```python
from build123d import *

# Parameters (mm, degrees)
SKETCH1_R           = 7.4
BOSS_EXTRUDE1_DEPTH = 6
SKETCH2_R           = 10
SKETCH2_R_2         = 1.5
BOSS_EXTRUDE2_DEPTH = 3
FILLET1_R           = 2.5


with BuildPart() as part:
    # Sketch1 → Boss-Extrude1 (new body)
    with BuildSketch(Plane(origin=(0, 0, 0), x_dir=(1, 0, 0), z_dir=(0, 1, 0))):
        with Locations(Location((0, 0, 0), (0, 0, 270))):
            Circle(SKETCH1_R)
        with BuildLine():
            Line((2.2, 2.219374912), (2.2, -2.219374912))
            ThreePointArc((2.2, -2.219374912), (-3.125, 0), (2.2, 2.219374912))
        make_face(mode=Mode.SUBTRACT)
    extrude(amount=BOSS_EXTRUDE1_DEPTH)

    # Sketch2 → Boss-Extrude2 (add)
    with BuildSketch(Plane(origin=(0, 6, 0), x_dir=(1, 0, 0), z_dir=(0, 1, 0))):
        with Locations(Location((0, 0, 0), (0, 0, 270))):
            Circle(SKETCH2_R)
        with Locations(Location((0, 0, 0), (0, 0, 270))):
            Circle(SKETCH2_R_2, mode=Mode.SUBTRACT)
    extrude(amount=BOSS_EXTRUDE2_DEPTH)

    # Fillet1
    fillet1_edges = [part.edges().sort_by_distance(p)[0] for p in [
        (0, 9, -10),
    ]]
    fillet(fillet1_edges, radius=FILLET1_R)


solid = part.part
```
The model under review builds one solid part; all positions refer to its coordinate system, in mm. A direction names the side the tool comes from. Round coordinates to 2 decimals unless told otherwise and drop trailing zeros. Order: outer loops, then holes, each group sorted by start corner. A loop starts at its lowest first (then second) coordinate and runs counter-clockwise, first axis right, second up. Notation, with made-up numbers: (63, -7) -> (75, -7) arc R14 cw to (75, 8) -> close; hole circle Ø6 at (22, 63.25). An arc over 180 degrees is marked (long way). One line per item, written item: value. Start each with the question number.
Q1. Mouldability with a two-part tool opening along X and no side actions: class faces 3 (the face through (0.45, 7.48, 1.43)), 4 (the face through (-3, 0, 2)), 5 (the face through (-9.76, 6.25, -2.17)) as released by +X, released by -X, zero draft, split by the parting line, or undercut.
Q2. Machinability: for faces 1 (the face through (0, 9, 2)), 2 (the face through (7.5, 6, 1.4)), which of the approach directions +Z, -Z, +X, -X, +Y, -Y give a long, thin tool a straight path to every point of the face, cutting with its end or side? Answer none if there is none.
Q3. Take a section at A-A (z = 0). Write out the cut boundary in (x, y) (3 decimals), and give its area (3 significant figures).
Q4. Clearance check with flat-ended pins moving along their axes: pin 1 Ø1.5 at (x, z) = (6, 5) entering from +Y; pin 2 Ø1.5 at (y, z) = (1, -0.5) entering from +X; pin 3 Ø5 at (x, y) = (-4, 2.5) entering from -Z; pin 4 Ø1.3 at (y, z) = (4, 1) entering from -X. State where each tip first meets the part, or that it passes through.
Q5. Wall thickness on line 1 (X direction, y = 2.3, z = 0) (3 decimals); line 2 (Y direction, x = 1.75, z = 1.25); line 3 (X direction, y = 6.8, z = 0): over which ranges is each line inside the solid? List them lowest first.
Q6. Take a section at D-D (y = 8.25). Write out the cut boundary in (x, z).
Q7. Take a section at B-B (x = 0). Write out the cut boundary in (y, z) (3 decimals).
Q8. Take a section at C-C (y = 5.5). Write out the cut boundary in (x, z) (3 decimals), and give its area (3 significant figures).
Reported:
1. face 3: undercut
1. face 4: zero draft
1. face 5: split by the parting line
2. face 1: +Z, -Z, +X, -X, +Y
2. face 2: -Y
3. outline: (-10, 6) -> (-7.4, 6) -> (-7.4, 0) -> (-3.125, 0) -> (-3.125, 6) -> (-1.5, 6) -> (-1.5, 9) -> (-7.5, 9) arc R2.5 ccw to (-10, 6.5) -> close; (1.5, 6) -> (2.2, 6) -> (2.2, 0) -> (7.4, 0) -> (7.4, 6) -> (10, 6) -> (10, 6.5) arc R2.5 ccw to (7.5, 9) -> (1.5, 9) -> close
3. area: 105 mm2
4. pin 1: stops at y = 9
4. pin 2: stops at x = 7.4
4. pin 3: stops at z = -7.25
4. pin 4: stops at x = -7.39
5. line 1: x = -7.4 to -3.125, 2.2 to 7.4
5. line 2: y = 6 to 9
5. line 3: x = -9.98 to -1.5, 1.5 to 9.98
6. outline: circle Ø18.57 at (0, 0); hole circle Ø3 at (0, 0)
7. outline: (0, -7.4) -> (6, -7.4) -> (6, -10) -> (6.5, -10) arc R2.5 ccw to (9, -7.5) -> (9, -1.5) -> (6, -1.5) -> (6, -3.125) -> (0, -3.125) -> close; (0, 3.125) -> (6, 3.125) -> (6, 1.5) -> (9, 1.5) -> (9, 7.5) arc R2.5 ccw to (6.5, 10) -> (6, 10) -> (6, 7.4) -> (0, 7.4) -> close
8. outline: circle Ø14.8 at (0, 0); hole (2.2, -2.219) -> (2.2, 2.219) arc R3.125 ccw (long way) to start
8. area: 144 mm2
